Here's how the part is built. I have some questions about the finished solid (model axes, mm). A direction names the side the tool comes from. Coordinates: 2 decimals unless noted, no trailing zeros. Write each loop counter-clockwise with the first axis right and the second up, starting at its lowest first coordinate (ties: lowest second). Pieces come first, ordered by that corner, then holes. Notation, with made-up numbers: (68, 73) - (75, 73) arc R13 ccw to (75, 95) - close; hole circle Ø11 at (-34, 18). An arc over 180 degrees is marked (long way). Answer in a Markdown table with one row per item. Add a question column.
Item 1: Which directions (+Z, -Z, +X, -X, +Y, -Y) give clear straight access to the entire face, cutting with the end or side of a thin tool? Please do faces 4 (the face through (-25, -2, 47.625)), 5 (the face through (40, -2, 44.45)), 6 (the face through (-40, -2, 12.7)), 7 (the face through (40, -2, -31.75)).
Item 2: We'd pull the mould along X, two halves only. Please class faces 1 (the face through (-41.275, -2, -38)), 2 (the face through (31.75, -2, 49)), 3 (the face through (40, -2, 25.4)): +X half, -X half, draft (parallel to the pull), parting line (faces both ways), or undercut.
Item 3: Imagine slicing it at A-A (z = -28). Please give me the cut outline in (x, y) (3 decimals), plus the area to 3 significant figures.
Item 4: I'm going to push flat-ended pins straight in: pin 1 (1.6 mm diameter, centred on x = 39, y = -2, fed in from -Z); pin 2 (1.6 mm diameter, centred on y = -1, z = -28, fed in from +X); pin 3 (1.6 mm diameter, centred on y = -2, z = -10, fed in from -X). Where does each tip first touch, or does it pass through?
Item 5: If I drill on probe 1 along X at (y, z) = (-0.95, -7.5); probe 2 along Z at (x, y) = (29.5, -2.15) (3 decimals), over which ranges is the centre line in solid material (lowest first)? Write a range as from..to.
Item 6: Imagine slicing it at B-B (x = 1). Please give me the cut outline in (y, z) (3 decimals), plus the area to 4 significant figures.
from build123d import *

# Parameters (mm, degrees)
F0_W     = 82.55
F0_H     = 101.6
F1_DEPTH = 3.175
F2_W     = 3.175
F2_H     = 6.35
F3_DEPTH = 3.176
F4_W     = 12.7
F4_H     = 3.175
F5_DEPTH = 3.176


with BuildPart() as f1:
    # F0 (on Front) → F1 (new body)
    with BuildSketch(Plane.XZ):
        Rectangle(F0_W, F0_H)
    extrude(amount=F1_DEPTH)

    # F2 (on face) → F3 (cut, through all)
    with BuildSketch(Plane.XZ.offset(3.175)):
        with Locations((-39.6875, -47.625)):
            Rectangle(F2_W, F2_H)
        with Locations((-39.6875, -28.575)):
            Rectangle(F2_W, F2_H)
        with Locations((-39.6875, -9.525)):
            Rectangle(F2_W, F2_H)
        with Locations((-39.6875, 9.525)):
            Rectangle(F2_W, F2_H)
        with Locations((-39.6875, 28.575)):
            Rectangle(F2_W, F2_H)
        with Locations((-39.6875, 47.625)):
            Rectangle(F2_W, F2_H)
        with Locations((39.6875, -47.625)):
            Rectangle(F2_W, F2_H)
        with Locations((39.6875, -9.525)):
            Rectangle(F2_W, F2_H)
        with Locations((39.6875, 9.525)):
            Rectangle(F2_W, F2_H)
        with Locations((39.6875, -28.575)):
            Rectangle(F2_W, F2_H)
        with Locations((39.6875, 28.575)):
            Rectangle(F2_W, F2_H)
        with Locations((39.6875, 47.625)):
            Rectangle(F2_W, F2_H)
    extrude(amount=-F3_DEPTH, mode=Mode.SUBTRACT)

    # F4 (on face) → F5 (cut, through all)
    with BuildSketch(Plane.XZ.offset(3.175)):
        with Locations((-25.4, 49.2125)):
            Rectangle(F4_W, F4_H)
        with Locations((0, 49.2125)):
            Rectangle(F4_W, F4_H)
        with Locations((25.4, 49.2125)):
            Rectangle(F4_W, F4_H)
    extrude(amount=-F5_DEPTH, mode=Mode.SUBTRACT)


solid = f1.part
Here are the results:
| question | item | result |
|---|---|---|
| 1 | face 4 | +Z, +Y, -Y |
| 1 | face 5 | +Z, +X, +Y, -Y |
| 1 | face 6 | -X, +Y, -Y |
| 1 | face 7 | +X, +Y, -Y |
| 2 | face 1 | -X half |
| 2 | face 2 | undercut |
| 2 | face 3 | draft |
| 3 | outline | (-38.1, -3.175) - (38.1, -3.175) - (38.1, 0) - (-38.1, 0) - close |
| 3 | area | 242 mm2 |
| 4 | pin 1 | stops at z = -44.45 |
| 4 | pin 2 | stops at x = 38.1 |
| 4 | pin 3 | stops at x = -38.1 |
| 5 | probe 1 | x = -38.1..38.1 |
| 5 | probe 2 | z = -50.8..47.625 |
| 6 | outline | (-3.175, -50.8) - (0, -50.8) - (0, 47.625) - (-3.175, 47.625) - close |
| 6 | area | 312.5 mm2 |
